Here's how the part is built. I have some questions about the finished solid (model axes, mm). Face numbers are marked on the shaded views. A direction names the side the tool comes from. Give positions to 0.01 mm unless a question says otherwise; leave off trailing zeros. Order: outer loops, then holes, each group sorted by start corner. A loop starts at its lowest first (then second) coordinate and runs counter-clockwise, first axis right, second up. Notation, with made-up numbers: (82.5, 74.25) -> (141.5, 74.25) arc R7 cw to (141.5, 82.25) -> close; hole circle Ø9 at (64.25, 68). An arc over 180 degrees is marked (long way). Write each question's results on one line, items separated by ' | '. Start each with the question number.
Q1. I'm going to push flat-ended pins straight in: pin 1 (4 mm diameter, centred on x = -7, y = -1, fed in from -Z); pin 2 (3 mm diameter, centred on x = -8, z = -0.5, fed in from -Y); pin 3 (1.5 mm diameter, centred on x = -2, z = 34, fed in from +Y). Where does each tip first touch, or does it pass through?
Q2. I need wall thicknesses on line 1 along Y through (x, z) = (14, 0); line 2 along X through (y, z) = (-19.5, -39.5); line 3 along Z through (x, y) = (-20, 35). Which ranges of each line are inside material? Lowest first, please. Write a range as [from, to].
Q3. Thinking about a two-plate mould opening in Z: for the marked faces 1, 2 and 3, which applies, pulls with the +Z half, pulls with the -Z half, needs draft (parallel to the pull), parting line crosses it, or undercut?
Q4. For the marked faces 4, 5 and 6, which set-ups out of +Z, -Z, +X, -X, +Y, -Y let a thin tool reach every point of the face, with its end or its side?
Q5. Imagine slicing it at A-A, the plane x = 2. Please give me the cut outline in (y, z).
Q6. Imagine slicing it at B-B, the plane x = 9. Please give me the cut outline in (y, z).
```python
from build123d import *

# Parameters (mm, degrees)
SKETCH1_R               = 57.15
BOSS_EXTRUDE1_DEPTH     = 6.35
SKETCH2_R               = 45.847
BOSS_EXTRUDE2_DEPTH     = 25.4
SKETCH11_R              = 1.89865
CUT_EXTRUDE3_DEPTH      = 10.16
CIRPATTERN1_COUNT       = 12
SKETCH15_R              = 5.55625
CUT_EXTRUDE4_DEPTH      = 1
CUT_EXTRUDE4_DEPTH_BACK = 32.7500001
SKETCH17_R              = 13.97
SKETCH17_R_2            = 5.55625
BOSS_EXTRUDE3_DEPTH     = 9.652
SKETCH18_R              = 38.354
CUT_EXTRUDE5_DEPTH      = 6.604
SKETCH19_R              = 1.1303
CUT_EXTRUDE6_DEPTH      = 6.35


with BuildPart() as part:
    # Sketch1 → Boss-Extrude1 (new body)
    with BuildSketch(Plane(origin=(0, 0, 0), x_dir=(0, 0, -1), z_dir=(1, 0, 0))):
        Circle(SKETCH1_R)
    extrude(amount=BOSS_EXTRUDE1_DEPTH)

    # Sketch2 → Boss-Extrude2 (add)
    with BuildSketch(Plane.ZY):
        Circle(SKETCH2_R)
    extrude(amount=BOSS_EXTRUDE2_DEPTH)

    # Sketch11 → Cut-Extrude3 (cut)
    with BuildSketch(Plane(origin=(0, 0, -45.847), x_dir=(-1, 0, 0), z_dir=(0, 0, -1))):
        with Locations((7.62, 0)):
            Circle(SKETCH11_R)
    cut_extrude3 = extrude(amount=-CUT_EXTRUDE3_DEPTH, mode=Mode.SUBTRACT)

    # CirPattern1: Cut-Extrude3 ×12 about axis
    cirpattern1_axis = Axis((0, 0, 0), (1, 0, 0))
    for i in range(1, CIRPATTERN1_COUNT):
        add(cut_extrude3.rotate(cirpattern1_axis, i * 360 / CIRPATTERN1_COUNT), mode=Mode.SUBTRACT)

    # Sketch15 → Cut-Extrude4 (cut, two sides)
    with BuildSketch(Plane(origin=(6.35, 0, 0), x_dir=(0, 0, -1), z_dir=(1, 0, 0))) as cut_extrude4_sk:
        Circle(SKETCH15_R)
    extrude(amount=CUT_EXTRUDE4_DEPTH, mode=Mode.SUBTRACT)
    extrude(cut_extrude4_sk.sketch, amount=-CUT_EXTRUDE4_DEPTH_BACK, mode=Mode.SUBTRACT)

    # Sketch16 → Cut-Revolve1 (revolve, cut)
    with BuildSketch(Plane.XY):
        with BuildLine():
            Line((-21.59, 45.847), (-14.4018, 45.847))
            Line((-14.4018, 45.847), (-14.4018, 44.069))
            ThreePointArc((-14.4018, 44.069), (-14.624984633, 43.530184633), (-15.1638, 43.307))
            Line((-15.1638, 43.307), (-20.828, 43.307))
            ThreePointArc((-20.828, 43.307), (-21.366815367, 43.530184633), (-21.59, 44.069))
            Line((-21.59, 44.069), (-21.59, 45.847))
        make_face()
    revolve(axis=Axis((0, 0, 0), (-1, 0, 0)), mode=Mode.SUBTRACT)

    # Sketch17 → Boss-Extrude3 (add)
    with BuildSketch(Plane(origin=(6.35, 0, 0), x_dir=(0, 0, -1), z_dir=(1, 0, 0))):
        Circle(SKETCH17_R)
        Circle(SKETCH17_R_2, mode=Mode.SUBTRACT)
    extrude(amount=BOSS_EXTRUDE3_DEPTH)

    # Sketch18 → Cut-Extrude5 (cut)
    with BuildSketch(Plane.ZY.offset(25.4)):
        Circle(SKETCH18_R)
    extrude(amount=-CUT_EXTRUDE5_DEPTH, mode=Mode.SUBTRACT)

    # Sketch19 → Cut-Extrude6 (cut)
    with BuildSketch(Plane.ZY.offset(18.796)):
        with Locations((0, 33.3375)):
            Circle(SKETCH19_R)
        with Locations((23.573172318, 23.573172318)):
            Circle(SKETCH19_R)
        with Locations((33.3375, 0)):
            Circle(SKETCH19_R)
        with Locations((23.573172318, -23.573172318)):
            Circle(SKETCH19_R)
        with Locations((0, -33.3375)):
            Circle(SKETCH19_R)
        with Locations((-23.573172318, -23.573172318)):
            Circle(SKETCH19_R)
        with Locations((-33.3375, 0)):
            Circle(SKETCH19_R)
        with Locations((-23.573172318, 23.573172318)):
            Circle(SKETCH19_R)
    extrude(amount=-CUT_EXTRUDE6_DEPTH, mode=Mode.SUBTRACT)

    # Sketch20 → Cut-Revolve2 (revolve, cut)
    with BuildSketch(Plane.XY):
        Polygon((0, 0), (-18.796, 0), (-18.796, 27.94), (0, 15.875), align=None)
    revolve(axis=Axis((0, 0, 0), (-1, 0, 0)), mode=Mode.SUBTRACT)


solid = part.part
```
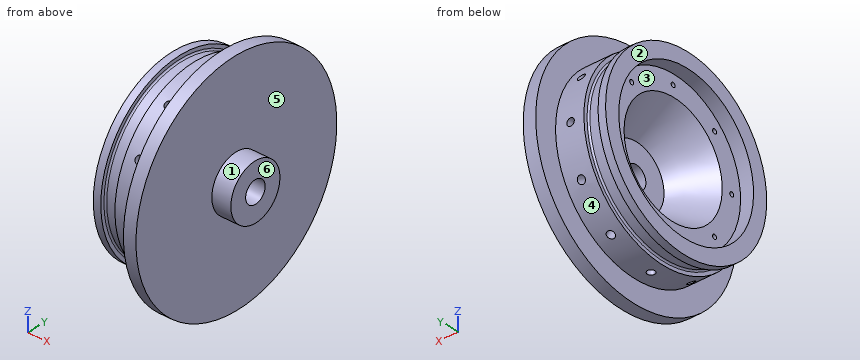
Geometry check:
1) pin 1: z = -45.85 | pin 2: y = -45.85 | pin 3: y = 31.57
2) line 1: [-13.97, -5.56], [5.56, 13.97] | line 2: [-25.4, -21.59], [-14.4, 6.35] | line 3: [-25.5, -15.69], [15.69, 25.5]
3) face 1: parting line crosses it | face 2: needs draft | face 3: undercut
4) face 4: -X | face 5: +X | face 6: +Z, -Z, +X, +Y, -Y
5) outline: circle Ø114.3 at (0, 0); hole circle Ø11.11 at (0, 0)
6) outline: circle Ø27.94 at (0, 0); hole circle Ø11.11 at (0, 0)
